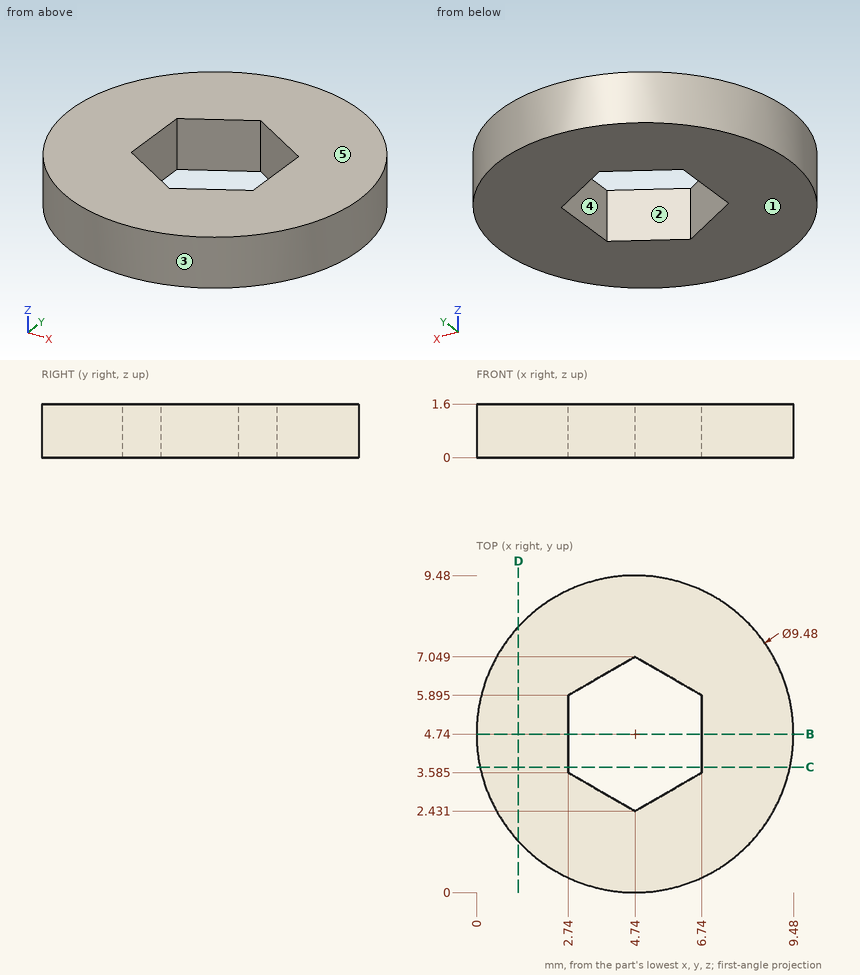
For this review, use the dimensioned drawing (mm, ordinates from the lowest corner) and the shaded views. A direction names the side the tool comes from. Give positions to 0.01 mm unless a question says otherwise; leave off trailing zeros. Order: outer loops, then holes, each group sorted by start corner. A loop starts at its lowest first (then second) coordinate and runs counter-clockwise, first axis right, second up. Notation, with made-up numbers: (81.5, 1) -> (131.5, 1) arc R24 ccw to (131.5, 25) -> close; hole circle Ø11 at (-4, 15). An arc over 180 degrees is marked (long way). Write item = value, one per line. Start each with the question number.
(1) For L1, parallel to Y at x = 4, z = 0.8; L2, parallel to X at y = 5.25, z = 0.75; L3, parallel to Y at x = 4.25, z = 1.3 (1 decimal), list the stretches that pass through material, from the lowest coordinate up. Write a range as from..to.
(2) Draft analysis for pull direction Y (two halves, no side actions). For the marked faces 1, 2 and 3, state which applies: +Y half, -Y half, draft (parallel to the pull), parting line (faces both ways), or undercut.
(3) Take a section at B-B (y = 4.74). Write out the cut boundary in (x, z).
(4) Take a section at D-D (x = 1.25). Write out the cut boundary in (y, z), plus the area to 3 significant figures.
(5) Take a section at C-C (y = 3.75). Write out the cut boundary in (x, z) (1 decimal).
(6) Tool access review of the marked faces 4 and 5: name each direction out of +Z, -Z, +X, -X, +Y, -Y from which nothing blocks a thin tool from reaching the whole face with its end or side.
Returned:
q1.L1 = 0.06..2.86, 6.62..9.42
q1.L2 = 0.03..2.74, 6.74..9.45
q1.L3 = 0..2.7, 6.8..9.5
q2.face_1 = draft
q2.face_2 = undercut
q2.face_3 = parting line
q3.outline = (0, 0) -> (2.74, 0) -> (2.74, 1.6) -> (0, 1.6) -> close; (6.74, 0) -> (9.48, 0) -> (9.48, 1.6) -> (6.74, 1.6) -> close
q4.outline = (1.53, 0) -> (7.95, 0) -> (7.95, 1.6) -> (1.53, 1.6) -> close
q4.area = 10.3 mm²
q5.outline = (0.1, 0) -> (2.7, 0) -> (2.7, 1.6) -> (0.1, 1.6) -> close; (6.7, 0) -> (9.4, 0) -> (9.4, 1.6) -> (6.7, 1.6) -> close
q6.face_4 = +Z, -Z
q6.face_5 = +Z, +X, -X, +Y, -Y
